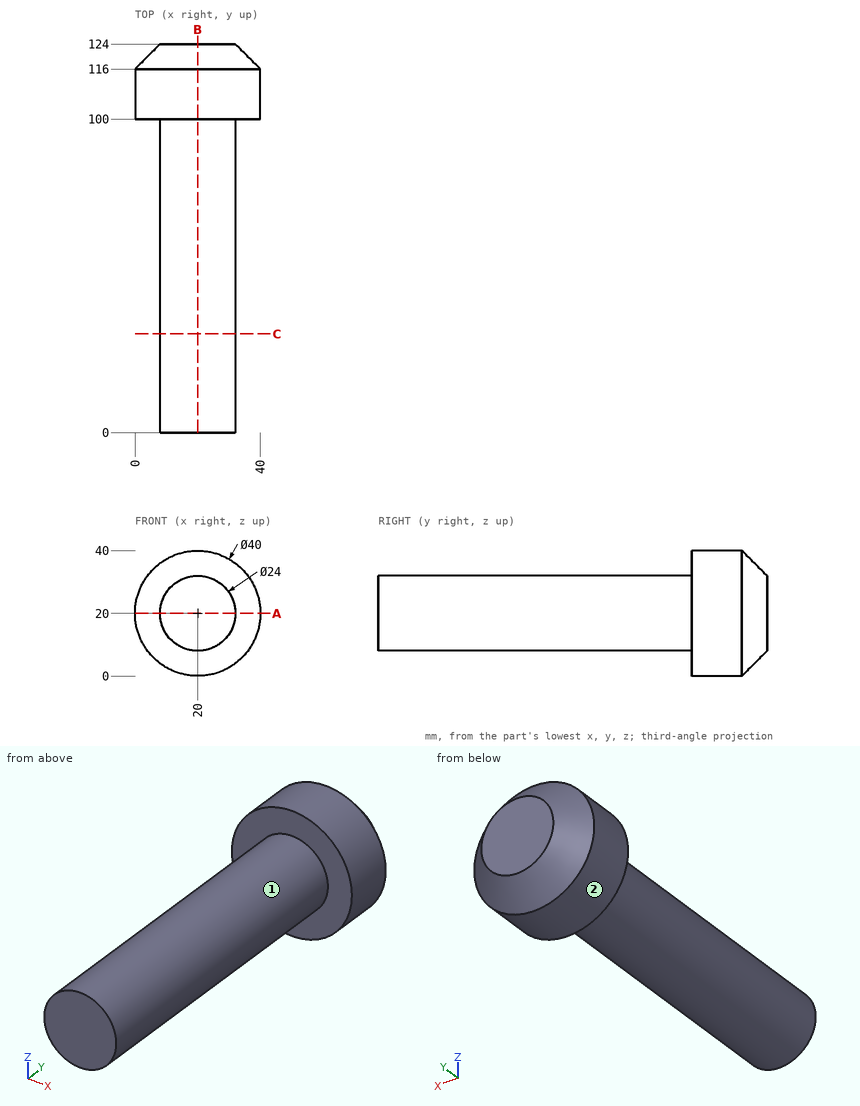
Design review of the part shown in the three views and the two pictorial views. Dimensions are in mm from the part's minimum x, y and z. A direction names the side the tool comes from. Give positions to 0.01 mm unless a question says otherwise; leave off trailing zeros. Order: outer loops, then holes, each group sorted by start corner. A loop starts at its lowest first (then second) coordinate and runs counter-clockwise, first axis right, second up. Notation, with made-up numbers: (73.25, 24.25) -> (105.25, 24.25) arc R20 ccw to (105.25, 33.25) -> close; hole circle Ø8 at (78.5, 17.5). An arc over 180 degrees is marked (long way). Write each question's results on one line, items separated by ' | '. Start each with the question number.
Q1. Wall thickness on L1, parallel to Y at x = 9.5, z = 28.5; L2, parallel to Y at x = 7, z = 34; L3, parallel to X at y = 40, z = 30: over which ranges is each line inside the solid? List them lowest first. Write a range as from..to.
Q2. Add section A-A on z = 20. Give the boundary of the cut face in (x, y).
Q3. Machinability: for the marked faces 1 and 2, which of the approach directions +Z, -Z, +X, -X, +Y, -Y give a long, thin tool a straight path to every point of the face, cutting with its end or side? Answer none if there is none.
Q4. For pin 1 (1.5 mm diameter, centred on x = 7, z = 10, fed in from -Y); pin 2 (1.5 mm diameter, centred on y = 54, z = 24, fed in from +X); pin 3 (3 mm diameter, centred on x = 25, y = 33.5, fed in from +Z), all flat-tipped, find the tip position at first contact; note any pin that passes through.
Q5. Add section C-C on y = 31.5. Give the boundary of the cut face in (x, z).
Q6. Add section B-B on x = 20. Give the boundary of the cut face in (y, z), and give its area (3 significant figures).
Found:
1) L1: y = 100..122.49 | L2: y = 100..116.9 | L3: x = 13.37..26.63
2) outline: (0, 100) -> (8, 100) -> (8, 0) -> (32, 0) -> (32, 100) -> (40, 100) -> (40, 116) -> (32, 124) -> (8, 124) -> (0, 116) -> close
3) face 1: -Y | face 2: +Y, -Y
4) pin 1: stops at y = 100 | pin 2: stops at x = 31.55 | pin 3: stops at z = 31.48
5) outline: circle Ø24 at (20, 20)
6) outline: (0, 8) -> (100, 8) -> (100, 0) -> (116, 0) -> (124, 8) -> (124, 32) -> (116, 40) -> (100, 40) -> (100, 32) -> (0, 32) -> close | area: 3,300 mm2
